Design review of the part built by this model. Coordinates are the model's own, in mm. Give positions to 0.01 mm unless a question says otherwise; leave off trailing zeros. Loops run counter-clockwise (first coordinate to the right, second up) from the corner with the lowest first, then second, coordinate; pieces in that order, holes last. Notation, with made-up numbers: (21, 25) -> (39, 25) arc R23 ccw to (39, 35) -> close; hole circle Ø2 at (15.25, 50.5). An arc over 180 degrees is marked (long way). Use CSV: the item, a comma, the result in double quotes. Start each with the question number.
Item 1: We need section B-B (z = -56.5). State the section outline as (x, y) points, plus the area to 3 significant figures.
Item 2: We need section D-D (z = 48). State the section outline as (x, y) points.
Item 3: We need section C-C (y = -15). Count the separate pieces of the cut face and the enclosed holes in it, plus the area to 3 significant figures.
Item 4: Wall thickness on line 1 along Z through (x, y) = (-39.5, -18.5); line 2 along Z through (x, y) = (166, -9.5): over which ranges is each line inside the solid? List them lowest first. Write a range as from..to.
Item 5: We need section A-A (x = 167). State the section outline as (y, z) points.
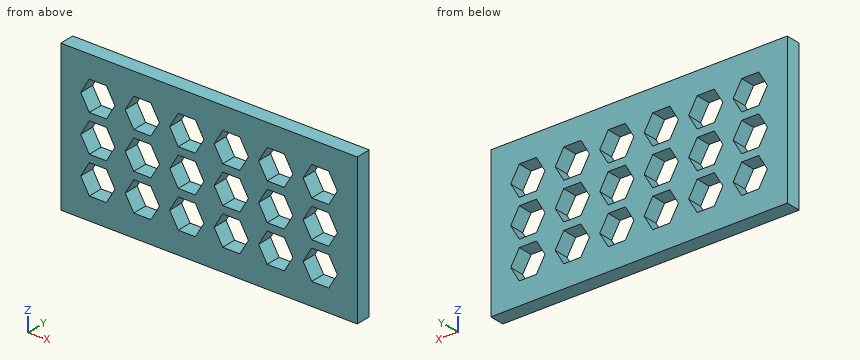
from build123d import *

# Parameters (mm, degrees)
F0_W     = 508
F0_H     = 254
F1_DEPTH = 25.4


with BuildPart() as f1:
    # F0 (on Front) → F1 (new body)
    with BuildSketch(Plane.XZ):
        Rectangle(F0_W, F0_H)
        Polygon((-161.170606, -63.5), (-175.835303, -88.9), (-205.164697, -88.9), (-219.829394, -63.5), (-205.164697, -38.1), (-175.835303, -38.1), align=None, mode=Mode.SUBTRACT)
        Polygon((-99.635303, -88.9), (-128.964697, -88.9), (-143.629394, -63.5), (-128.964697, -38.1), (-99.635303, -38.1), (-84.970606, -63.5), align=None, mode=Mode.SUBTRACT)
        Polygon((-67.429394, -63.5), (-52.764697, -38.1), (-23.435303, -38.1), (-8.770606, -63.5), (-23.435303, -88.9), (-52.764697, -88.9), align=None, mode=Mode.SUBTRACT)
        Polygon((52.764697, -88.9), (23.435303, -88.9), (8.770606, -63.5), (23.435303, -38.1), (52.764697, -38.1), (67.429394, -63.5), align=None, mode=Mode.SUBTRACT)
        Polygon((128.964697, -38.1), (143.629394, -63.5), (128.964697, -88.9), (99.635303, -88.9), (84.970606, -63.5), (99.635303, -38.1), align=None, mode=Mode.SUBTRACT)
        Polygon((205.164697, -88.9), (175.835303, -88.9), (161.170606, -63.5), (175.835303, -38.1), (205.164697, -38.1), (219.829394, -63.5), align=None, mode=Mode.SUBTRACT)
        Polygon((-161.170606, 0), (-175.835303, -25.4), (-205.164697, -25.4), (-219.829394, 0), (-205.164697, 25.4), (-175.835303, 25.4), align=None, mode=Mode.SUBTRACT)
        Polygon((-99.635303, -25.4), (-128.964697, -25.4), (-143.629394, 0), (-128.964697, 25.4), (-99.635303, 25.4), (-84.970606, 0), align=None, mode=Mode.SUBTRACT)
        Polygon((-67.429394, 0), (-52.764697, 25.4), (-23.435303, 25.4), (-8.770606, 0), (-23.435303, -25.4), (-52.764697, -25.4), align=None, mode=Mode.SUBTRACT)
        Polygon((-175.835303, 88.9), (-161.170606, 63.5), (-175.835303, 38.1), (-205.164697, 38.1), (-219.829394, 63.5), (-205.164697, 88.9), align=None, mode=Mode.SUBTRACT)
        Polygon((-99.635303, 88.9), (-84.970606, 63.5), (-99.635303, 38.1), (-128.964697, 38.1), (-143.629394, 63.5), (-128.964697, 88.9), align=None, mode=Mode.SUBTRACT)
        Polygon((-23.435303, 88.9), (-8.770606, 63.5), (-23.435303, 38.1), (-52.764697, 38.1), (-67.429394, 63.5), (-52.764697, 88.9), align=None, mode=Mode.SUBTRACT)
        Polygon((52.764697, -25.4), (23.435303, -25.4), (8.770606, 0), (23.435303, 25.4), (52.764697, 25.4), (67.429394, 0), align=None, mode=Mode.SUBTRACT)
        Polygon((128.964697, 25.4), (143.629394, 0), (128.964697, -25.4), (99.635303, -25.4), (84.970606, 0), (99.635303, 25.4), align=None, mode=Mode.SUBTRACT)
        Polygon((205.164697, -25.4), (175.835303, -25.4), (161.170606, 0), (175.835303, 25.4), (205.164697, 25.4), (219.829394, 0), align=None, mode=Mode.SUBTRACT)
        Polygon((52.764697, 88.9), (67.429394, 63.5), (52.764697, 38.1), (23.435303, 38.1), (8.770606, 63.5), (23.435303, 88.9), align=None, mode=Mode.SUBTRACT)
        Polygon((128.964697, 88.9), (143.629394, 63.5), (128.964697, 38.1), (99.635303, 38.1), (84.970606, 63.5), (99.635303, 88.9), align=None, mode=Mode.SUBTRACT)
        Polygon((205.164697, 88.9), (219.829394, 63.5), (205.164697, 38.1), (175.835303, 38.1), (161.170606, 63.5), (175.835303, 88.9), align=None, mode=Mode.SUBTRACT)
    extrude(amount=F1_DEPTH)


solid = f1.part
Results found:
1,outline,"(-254, -25.4) -> (-215.79, -25.4) -> (-215.79, 0) -> (-254, 0) -> close; (-165.21, -25.4) -> (-139.59, -25.4) -> (-139.59, 0) -> (-165.21, 0) -> close; (-89.01, -25.4) -> (-63.39, -25.4) -> (-63.39, 0) -> (-89.01, 0) -> close; (-12.81, -25.4) -> (12.81, -25.4) -> (12.81, 0) -> (-12.81, 0) -> close; (63.39, -25.4) -> (89.01, -25.4) -> (89.01, 0) -> (63.39, 0) -> close; (139.59, -25.4) -> (165.21, -25.4) -> (165.21, 0) -> (139.59, 0) -> close; (215.79, -25.4) -> (254, -25.4) -> (254, 0) -> (215.79, 0) -> close"
1,area,"5,200 mm²"
2,outline,"(-254, -25.4) -> (-210.88, -25.4) -> (-210.88, 0) -> (-254, 0) -> close; (-170.12, -25.4) -> (-134.68, -25.4) -> (-134.68, 0) -> (-170.12, 0) -> close; (-93.92, -25.4) -> (-58.48, -25.4) -> (-58.48, 0) -> (-93.92, 0) -> close; (-17.72, -25.4) -> (17.72, -25.4) -> (17.72, 0) -> (-17.72, 0) -> close; (58.48, -25.4) -> (93.92, -25.4) -> (93.92, 0) -> (58.48, 0) -> close; (134.68, -25.4) -> (170.12, -25.4) -> (170.12, 0) -> (134.68, 0) -> close; (210.88, -25.4) -> (254, -25.4) -> (254, 0) -> (210.88, 0) -> close"
3,separate pieces,"1"
3,enclosed holes,"18"
3,area,"88,800 mm²"
4,line 1,"-127..-88.9, -38.1..-25.4, 25.4..38.1, 88.9..127"
4,line 2,"-127..-71.86, -55.14..-8.36, 8.36..55.14, 71.86..127"
5,outline,"(-25.4, -127) -> (0, -127) -> (0, -73.6) -> (-25.4, -73.6) -> close; (-25.4, -53.4) -> (0, -53.4) -> (0, -10.1) -> (-25.4, -10.1) -> close; (-25.4, 10.1) -> (0, 10.1) -> (0, 53.4) -> (-25.4, 53.4) -> close; (-25.4, 73.6) -> (0, 73.6) -> (0, 127) -> (-25.4, 127) -> close"
